```python
from build123d import *

# Parameters (mm, degrees)
CROQUIS1_W              = 110
CROQUIS1_H              = 110
CROQUIS1_W_2            = 75
CROQUIS1_H_2            = 75
SALIENTE_EXTRUIR1_DEPTH = 6.5
CROQUIS2_W              = 140
CROQUIS2_H              = 140
CROQUIS2_R              = 3.5
CROQUIS2_R_2            = 2.5
SALIENTE_EXTRUIR2_DEPTH = 6.5


with BuildPart() as part:
    # Croquis1 → Saliente-Extruir1 (new body)
    with BuildSketch(Plane(origin=(0, 0, 0), x_dir=(1, 0, 0), z_dir=(0, 1, 0))):
        with Locations((55, 55)):
            Rectangle(CROQUIS1_W, CROQUIS1_H)
        with Locations((55, 55)):
            Rectangle(CROQUIS1_W_2, CROQUIS1_H_2, mode=Mode.SUBTRACT)
    extrude(amount=SALIENTE_EXTRUIR1_DEPTH)

    # Croquis2 → Saliente-Extruir2 (add)
    with BuildSketch(Plane(origin=(0, 6.5, 0), x_dir=(1, 0, 0), z_dir=(0, 1, 0))):
        with Locations((55, 55)):
            Rectangle(CROQUIS2_W, CROQUIS2_H)
        with Locations(Location((55, 55, 0), (0, 0, 90))):
            Circle(CROQUIS2_R, mode=Mode.SUBTRACT)
        with Locations(Location((25, 85, 0), (0, 0, 90))):
            Circle(CROQUIS2_R_2, mode=Mode.SUBTRACT)
        with Locations(Location((85, 85, 0), (0, 0, 90))):
            Circle(CROQUIS2_R_2, mode=Mode.SUBTRACT)
        with Locations(Location((85, 25, 0), (0, 0, 90))):
            Circle(CROQUIS2_R_2, mode=Mode.SUBTRACT)
        with Locations(Location((25, 25, 0), (0, 0, 90))):
            Circle(CROQUIS2_R_2, mode=Mode.SUBTRACT)
        with Locations(Location((55, 85, 0), (0, 0, 90))):
            Circle(CROQUIS2_R_2, mode=Mode.SUBTRACT)
        with Locations(Location((85, 55, 0), (0, 0, 90))):
            Circle(CROQUIS2_R_2, mode=Mode.SUBTRACT)
        with Locations(Location((55, 25, 0), (0, 0, 90))):
            Circle(CROQUIS2_R_2, mode=Mode.SUBTRACT)
        with Locations(Location((25, 55, 0), (0, 0, 90))):
            Circle(CROQUIS2_R_2, mode=Mode.SUBTRACT)
    extrude(amount=SALIENTE_EXTRUIR2_DEPTH)


solid = part.part
```
Geometry: final body of the model. Coordinates: model frame, mm. A direction names the side the tool comes from. Give positions to 0.01 mm unless a question says otherwise; leave off trailing zeros. Order: outer loops, then holes, each group sorted by start corner. A loop starts at its lowest first (then second) coordinate and runs counter-clockwise, first axis right, second up. Notation, with made-up numbers: (63.25, 69.25) -> (100.25, 69.25) arc R21 cw to (100.25, 81.25) -> close; hole circle Ø3 at (-20.5, 72.5). An arc over 180 degrees is marked (long way). Write each question's results on one line, items separated by ' | '. Start each with the question number.
1) Draft query along X for faces 1 (the flat face through (0, 3, -54)), 2 (the flat face through (54, 3, -110)), 3 (the cylindrical face through (82.52, 9.7, -24.67)). Return one class per face: pulls with the +X half, pulls with the -X half, needs draft (parallel to the pull), parting line crosses it, or undercut.
2) Section C-C (y = 4). Return loops of the section in (x, z), then the cut area to 4 significant figures.
3) Section A-A (z = -55). Return loops of the section in (x, y).
4) Section D-D (x = 49.5). Return loops of the section in (y, z), then the cut area to 3 significant figures.
5) Set-up query: faces 4 (the flat face through (103, 0, -56)), 5 (the flat face through (54, 3, 0)), 6 (the flat face through (92.5, 3, -54)). Return all of +Z, -Z, +X, -X, +Y, -Y with unobstructed straight access to the full face (end or side cutting, diameter ignored); none if empty.
6) First-contact query: pin 1 (7 mm diameter, centred on x = 61.5, y = 1.5, fed in from -Z); pin 2 (2 mm diameter, centred on y = 4, z = -53, fed in from +X); pin 3 (5 mm diameter, centred on x = 58, z = -25.5, fed in from -Y). Flat tips, straight axial feed; report the tip coordinate or a pass-through.
7) Section B-B (x = 85). Return loops of the section in (y, z).
8) Line query: line 1 (X direction, y = 10.75, z = -55); line 2 (Z direction, x = 55, y = 8.75); line 3 (Z direction, x = 25, y = 8.75). Output: solid intervals per line, ascending. Write a range as from..to.
Calculated:
1) face 1: pulls with the -X half | face 2: needs draft | face 3: undercut
2) outline: (0, -110) -> (110, -110) -> (110, 0) -> (0, 0) -> close; hole (17.5, -92.5) -> (92.5, -92.5) -> (92.5, -17.5) -> (17.5, -17.5) -> close | area: 6,475 mm2
3) outline: (-15, 6.5) -> (0, 6.5) -> (0, 0) -> (17.5, 0) -> (17.5, 6.5) -> (22.5, 6.5) -> (22.5, 13) -> (-15, 13) -> close; (27.5, 6.5) -> (51.5, 6.5) -> (51.5, 13) -> (27.5, 13) -> close; (58.5, 6.5) -> (82.5, 6.5) -> (82.5, 13) -> (58.5, 13) -> close; (87.5, 6.5) -> (92.5, 6.5) -> (92.5, 0) -> (110, 0) -> (110, 6.5) -> (125, 6.5) -> (125, 13) -> (87.5, 13) -> close
4) outline: (0, -110) -> (6.5, -110) -> (6.5, -125) -> (13, -125) -> (13, 15) -> (6.5, 15) -> (6.5, 0) -> (0, 0) -> (0, -17.5) -> (6.5, -17.5) -> (6.5, -92.5) -> (0, -92.5) -> close | area: 1,140 mm2
5) face 4: +Z, -Z, +X, -X, -Y | face 5: +Z, +X, -X, -Y | face 6: -Y
6) pin 1: z = -110 | pin 2: x = 110 | pin 3: y = 6.5
7) outline: (0, -110) -> (6.5, -110) -> (6.5, -125) -> (13, -125) -> (13, -87.5) -> (6.5, -87.5) -> (6.5, -92.5) -> (0, -92.5) -> close; (0, -17.5) -> (6.5, -17.5) -> (6.5, -22.5) -> (13, -22.5) -> (13, 15) -> (6.5, 15) -> (6.5, 0) -> (0, 0) -> close; (6.5, -82.5) -> (13, -82.5) -> (13, -57.5) -> (6.5, -57.5) -> close; (6.5, -52.5) -> (13, -52.5) -> (13, -27.5) -> (6.5, -27.5) -> close
8) line 1: -15..22.5, 27.5..51.5, 58.5..82.5, 87.5..125 | line 2: -125..-87.5, -82.5..-58.5, -51.5..-27.5, -22.5..15 | line 3: -125..-87.5, -82.5..-57.5, -52.5..-27.5, -22.5..15
